Part model, mm, in its own coordinate system. A direction names the side the tool comes from. Give positions to 0.01 mm unless a question says otherwise; leave off trailing zeros.
from build123d import *

# Parameters (mm, degrees)
EXTRUDE_1_DEPTH     = 75
CUT_EXTRUDE_2_DEPTH = 89
CUT_EXTRUDE_3_DEPTH = 89
CUT_EXTRUDE_4_DEPTH = 102
FILLET_1_R          = 4
SKETCH_8_R          = 1.7
CUT_EXTRUDE_5_DEPTH = 27
SKETCH_9_R          = 3.1
CUT_EXTRUDE_6_DEPTH = 19.5


with BuildPart() as part:
    # 草图1 → 凸台-拉伸1 (new body)
    with BuildSketch(Plane(origin=(-39.59611161, -89.310119263, 1121.416485544), x_dir=(-0.9993811405079087, 0.0027925735986707154, -0.035064761938558196), z_dir=(0.03517578708588839, 0.07933995566829549, -0.9962267991965691))):
        with BuildLine():
            Line((-262.075571521, 359.155993571), (-261.628696205, 364.135983777))
            Line((-261.628696205, 364.135983777), (-261.435860549, 366.284949367))
            ThreePointArc((-261.435860549, 366.284949367), (-261.109064157, 368.074809297), (-260.463371375, 369.775831132))
            Line((-260.463371375, 369.775831132), (-248.776723549, 393.730780012))
            ThreePointArc((-248.776723549, 393.730780012), (-256.744007891, 423.508755886), (-287.342992795, 419.779467775))
            Line((-287.342992795, 419.779467775), (-315.661768776, 388.401500241))
            ThreePointArc((-315.661768776, 388.401500241), (-319.142063417, 383.007701172), (-320.734355269, 376.78917033))
            Line((-320.734355269, 376.78917033), (-321.388578677, 369.498487569))
            Line((-321.388578677, 369.498487569), (-321.835453993, 364.518497363))
            Line((-321.835453993, 364.518497363), (-262.075571521, 359.155993571))
        make_face()
    extrude(amount=EXTRUDE_1_DEPTH)

    # 草图2 → 切除-拉伸2 (cut)
    with BuildSketch(Plane(origin=(351.495487401, 30.478889762, 14.83831212), x_dir=(0.04186275100976059, 0.0036300044207880334, -0.999116776531052), z_dir=(0.995381658359661, 0.08631157133879107, 0.04201983881692256))):
        with BuildLine():
            Line((-1054.940506582, 279.262299259), (-1060.282877118, 349.349088516))
            Line((-1060.282877118, 349.349088516), (-1174.950235928, 340.60856087))
            Line((-1174.950235928, 340.60856087), (-1169.607865392, 270.521771613))
            Line((-1169.607865392, 270.521771613), (-1168.694349481, 258.537317011))
            Line((-1168.694349481, 258.537317011), (-1168.137997642, 251.238513271))
            ThreePointArc((-1168.137997642, 251.238513271), (-1159.493263254, 234.16850768), (-1141.310196239, 228.210941279))
            Line((-1141.310196239, 228.210941279), (-1076.498210824, 233.151239514))
            ThreePointArc((-1076.498210824, 233.151239514), (-1059.428205233, 241.795973902), (-1053.470638832, 259.979040917))
            Line((-1053.470638832, 259.979040917), (-1054.026990671, 267.277844657))
            Line((-1054.026990671, 267.277844657), (-1054.940506582, 279.262299259))
        make_face()
        with BuildLine():
            Line((-1075.381209674, 277.7042052), (-1079.165486151, 327.350291365))
            Line((-1079.165486151, 327.350291365), (-1152.951438777, 321.725951836))
            Line((-1152.951438777, 321.725951836), (-1149.1671623, 272.079865671))
            Line((-1149.1671623, 272.079865671), (-1148.253646388, 260.095411069))
            Line((-1148.253646388, 260.095411069), (-1147.69729455, 252.79660733))
            ThreePointArc((-1147.69729455, 252.79660733), (-1146.14124236, 249.724006324), (-1142.868290297, 248.651644371))
            Line((-1142.868290297, 248.651644371), (-1078.056304883, 253.591942606))
            ThreePointArc((-1078.056304883, 253.591942606), (-1074.983703877, 255.147994796), (-1073.911341925, 258.420946859))
            Line((-1073.911341925, 258.420946859), (-1074.467693763, 265.719750598))
            Line((-1074.467693763, 265.719750598), (-1075.381209674, 277.7042052))
        make_face(mode=Mode.SUBTRACT)
    extrude(amount=-CUT_EXTRUDE_2_DEPTH, mode=Mode.SUBTRACT)

    # 草图4 → 切除-拉伸3 (cut)
    with BuildSketch(Plane(origin=(-39.578523717, -89.270449285, 1120.918372145), x_dir=(0.9993811405079086, -0.002792573598663483, 0.03506476193856097), z_dir=(-0.03517578708589058, -0.0793399556682715, 0.9962267991965709))):
        with BuildLine():
            Line((273.293580359, 366.186740579), (261.539321142, 365.131981818))
            Line((261.539321142, 365.131981818), (235.445654793, 362.790488178))
            Line((235.445654793, 362.790488178), (232.049402391, 400.638413743))
            ThreePointArc((232.049402391, 400.638413743), (294.258339674, 433.19870407), (273.293580359, 366.186740579))
        make_face()
    extrude(amount=-CUT_EXTRUDE_3_DEPTH, mode=Mode.SUBTRACT)

    # 草图7 → 切除-拉伸4 (cut)
    with BuildSketch(Plane(origin=(-39.578523717, -89.270449285, 1120.918372145), x_dir=(0.9993811405079086, -0.002792573598663483, 0.03506476193856097), z_dir=(-0.03517578708589058, -0.0793399556682715, 0.996226799196571))):
        Polygon((303.866510818, 387.002501991), (315.940576228, 388.085958298), (314.335988901, 405.967521421), (302.261923491, 404.884065114), align=None)
    extrude(amount=-CUT_EXTRUDE_4_DEPTH, mode=Mode.SUBTRACT)

    # 圆角1
    fillet_1_edges = [part.edges().sort_by_distance(p)[0] for p in [
        (265.401440549, 298.597567558, 1125.436762489),
    ]]
    fillet(fillet_1_edges, radius=FILLET_1_R)

    # 草图8 → 切除-拉伸5 (cut)
    with BuildSketch(Plane(origin=(-29.90386421, 332.486882621, 25.423530653), x_dir=(0.9960030029050818, 0.0890597720529966, 0.0068099343556353885), z_dir=(0.08931975259739458, -0.9931039643902253, -0.07593745919082608))):
        with Locations(Location((277.335448654, 1110.342499925, 0), (0, 0, 359.608686584))):
            Circle(SKETCH_8_R)
        with Locations(Location((297.985718495, 1099.373618692, 0), (0, 0, 359.608686584))):
            Circle(SKETCH_8_R)
        with Locations(Location((278.161253776, 1086.974401032, 0), (0, 0, 359.608686584))):
            Circle(SKETCH_8_R)
    extrude(amount=-CUT_EXTRUDE_5_DEPTH, mode=Mode.SUBTRACT)

    # 草图9 → 切除-拉伸6 (cut)
    with BuildSketch(Plane(origin=(-32.002878396, 355.824825784, 27.208060944), x_dir=(0.9960030029050824, 0.08905977205298932, 0.006809934355638229), z_dir=(-0.08931975259738754, 0.9931039643902232, 0.07593745919086373))):
        with Locations(Location((278.161253776, -1086.974401032, 0), (0, 0, 180.391313416))):
            Circle(SKETCH_9_R)
        with Locations(Location((297.985718495, -1099.373618692, 0), (0, 0, 258.436796429))):
            Circle(SKETCH_9_R)
        with Locations(Location((277.335448654, -1110.342499925, 0), (0, 0, 180.391313416))):
            Circle(SKETCH_9_R)
    extrude(amount=-CUT_EXTRUDE_6_DEPTH, mode=Mode.SUBTRACT)


solid = part.part
1) 3-axis set-ups, long thin cutter, end or side, ignore diameter. For faces 4 (the flat face through (253.855, 274.042, 1123.53)), 5 (the flat face through (245.45, 278.34, 1110.1)): which of +Z, -Z, +X, -X, +Y, -Y reach the whole face in a straight line?
Check result:
face 4: -Z, +X, -Y
face 5: none
2) Mould opens along X. For faces 1 (the flat face through (229.04, 277.39, 1122.98)), 2 (the cylindrical face through (280.7, 294.42, 1126.16)), 3 (the flat face through (264.97, 278.96, 1124.96)) say: +X half, -X half, draft (parallel to the pull), parting line (faces both ways), or undercut.
Check result:
face 1: -X half
face 2: +X half
face 3: undercut
3) Flat gauge pins, fed straight in: P1, Ø4, axis at x = 236.5, z = 1100.5, coming from the -Y side; P2, Ø8, axis at y = 294, z = 1138.5, coming from the -X side; P3, Ø3, axis at x = 264.5, y = 282, coming from the -Z side. Where does each tip first touch, or does it go through?
Check result:
P1: stops at y = 274.01
P2: stops at x = 259.94
P3: stops at z = 1086.89
4) Drill centre lines: L1, parallel to Y at x = 235.5, z = 1102.5; L2, parallel to X at y = 285, z = 1152.5; L3, parallel to Y at x = 257.5, z = 1127.5. Where is each one in solid material? Low to high.
Check result:
L1: y = 274 to 279.54
L2: x = 255.64 to 281.4
L3: y = 274.07 to 287.88
